Check sheet for the drawn part. Datum: minimum x, y, z corner. Units: mm. Give positions to 0.01 mm unless a question says otherwise; leave off trailing zeros. Order: outer loops, then holes, each group sorted by start corner. A loop starts at its lowest first (then second) coordinate and runs counter-clockwise, first axis right, second up. Notation, with made-up numbers: (0, -3.5) -> (9, -3.5) arc R33 ccw to (9, 34.5) -> close; hole circle Ø5 at (15, 72). An arc over 180 degrees is marked (long way). Answer in a Markdown table with one row per item. Add a question column.
(1) Cross-section at D-D (x = 220). Record the cut outline in (y, z), then the cut area to 3 significant figures.
(2) Cross-section at C-C (z = 192). Record the cut outline in (x, y).
(3) Go/stop test with flat-tipped pins: pin 1 (7 mm diameter, centred on x = 234.5, y = 13.5, fed in from -Z); pin 2 (7.5 mm diameter, centred on y = 16, z = 162.5, fed in from +X). Record where each tip stops, or that it passes through.
(4) Cross-section at B-B (x = 71). Record the cut outline in (y, z).
(5) Release check for a two-part mould opening along Z. For the marked faces 1 and 2 record: released by +Z, released by -Z, zero draft, split by the parting line, or undercut.
(6) Thickness scan on L1, parallel to Z at x = 12, y = 21; L2, parallel to Z at x = 220, y = 18.25; L3, parallel to X at y = 7.25, z = 216. Record the ranges inside material, lowest first. Write a range as [from, to].
(7) Cross-section at A-A (y = 5.5). Record the cut outline in (x, z).
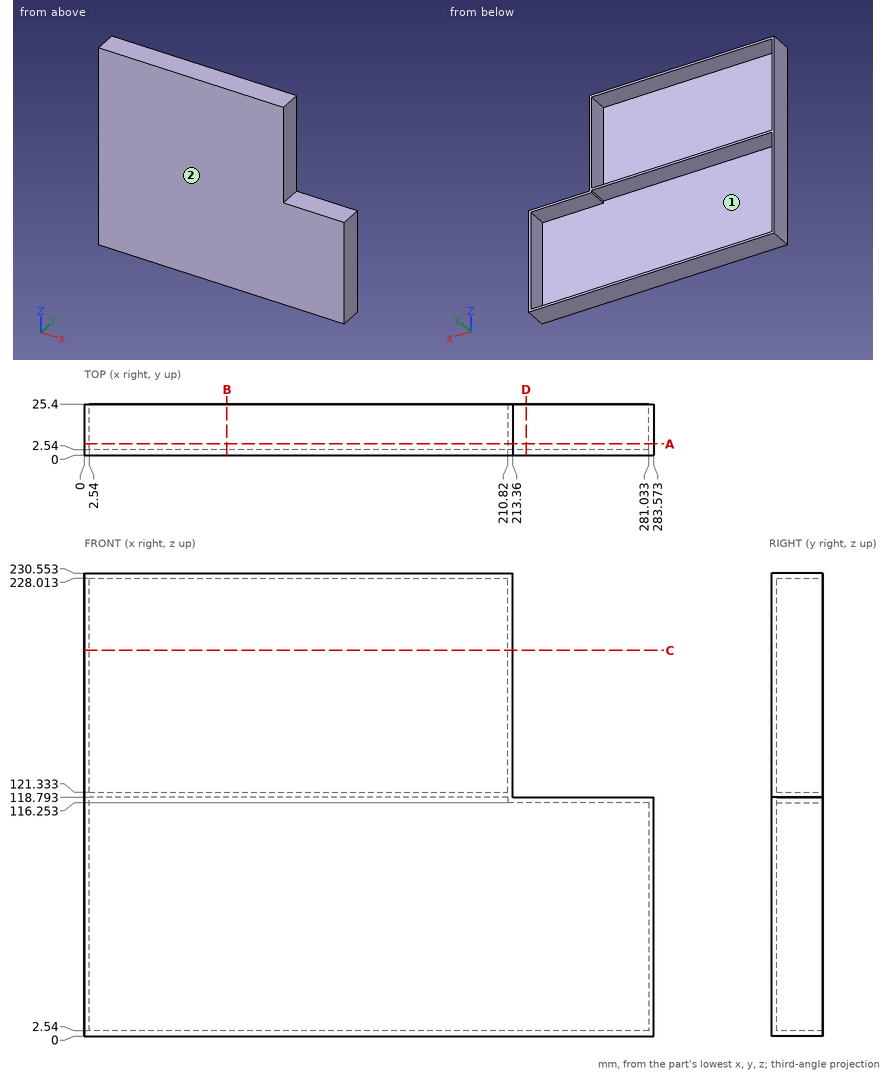
Answer below:
| question | item | result |
|---|---|---|
| 1 | outline | (0, 0) -> (25.4, 0) -> (25.4, 2.54) -> (2.54, 2.54) -> (2.54, 116.25) -> (25.4, 116.25) -> (25.4, 118.79) -> (0, 118.79) -> close |
| 1 | area | 418 mm² |
| 2 | outline | (0, 0) -> (213.36, 0) -> (213.36, 25.4) -> (210.82, 25.4) -> (210.82, 2.54) -> (2.54, 2.54) -> (2.54, 25.4) -> (0, 25.4) -> close |
| 3 | pin 1 | stops at z = 0 |
| 3 | pin 2 | stops at x = 213.36 |
| 4 | outline | (0, 0) -> (25.4, 0) -> (25.4, 2.54) -> (2.54, 2.54) -> (2.54, 118.79) -> (25.4, 118.79) -> (25.4, 121.33) -> (2.54, 121.33) -> (2.54, 228.01) -> (25.4, 228.01) -> (25.4, 230.55) -> (0, 230.55) -> close |
| 5 | face 1 | undercut |
| 5 | face 2 | zero draft |
| 6 | L1 | z = [0, 2.54], [118.79, 121.33], [228.01, 230.55] |
| 6 | L2 | z = [0, 2.54], [116.25, 118.79] |
| 6 | L3 | x = [0, 2.54], [210.82, 213.36] |
| 7 | outline | (0, 0) -> (283.57, 0) -> (283.57, 118.79) -> (213.36, 118.79) -> (213.36, 230.55) -> (0, 230.55) -> close; hole (2.54, 2.54) -> (281.03, 2.54) -> (281.03, 116.25) -> (210.82, 116.25) -> (210.82, 118.79) -> (2.54, 118.79) -> close; hole (2.54, 121.33) -> (210.82, 121.33) -> (210.82, 228.01) -> (2.54, 228.01) -> close |
